Build history of the part. All positions in model axes, mm. Face numbers are marked on the shaded views. Round coordinates to 2 decimals unless told otherwise and drop trailing zeros. Loops run counter-clockwise (first coordinate to the right, second up) from the corner with the lowest first, then second, coordinate; pieces in that order, holes last. Notation, with made-up numbers: (-28, 55.25) - (8, 55.25) arc R37 ccw to (8, 91.25) - close; hole circle Ø4 at (-9, -22.75). An arc over 180 degrees is marked (long way). Use one line per item in the form item = value. Start each with the question number.
Q1. Mould opens along Z. For the marked faces 1, 2 and 3 say: released by +Z, released by -Z, zero draft, split by the parting line, or undercut.
Q2. Drill centre lines: line 1 (Z direction, x = 18.75, y = 0); line 2 (Z direction, x = 11, y = 4.75); line 3 (X direction, y = -10.5, z = -2.5). Where is each one in solid material? Low to high.
Q3. Pin check, flat tips, straight feed: pin 1 (4 mm diameter, centred on x = 5.5, z = 3.5, fed in from +Y); pin 2 (1 mm diameter, centred on x = 21, y = 0.5, fed in from -Z); pin 3 (4 mm diameter, centred on x = 5.5, y = -3.5, fed in from +Z); pin 4 (7.5 mm diameter, centred on y = -6, z = -2.5, fed in from +X). Stop position of each tip, or through.
Q4. Saw through at A-A (z = 0). Give the cut face in (x, y), then the cut area to 3 significant figures.
Q5. Saw through at C-C (x = 11.5). Give the cut face in (y, z).
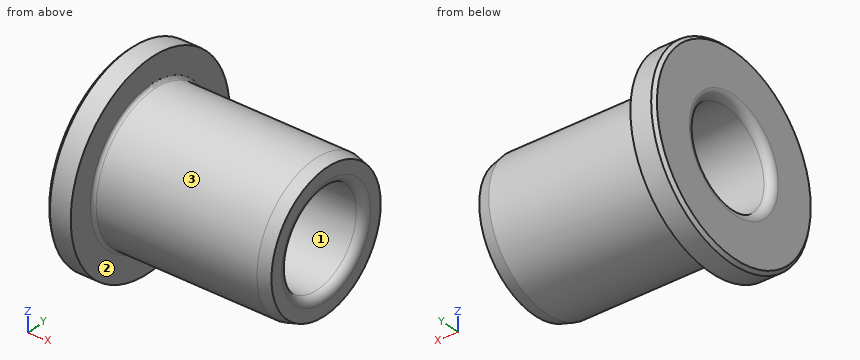
Autodesk Inventor part; units mm, degrees
ref_plane "YZ Plane" through (0, 0, 0) normal (1, 0, 0) x (0, 1, 0)
ref_plane "XZ Plane" through (0, 0, 0) normal (0, 1, 0) x (-1, 0, 0)
ref_plane "XY Plane" through (0, 0, 0) normal (0, 0, 1) x (1, 0, 0)
sketch "Sketch_1" plane through (0, 0, 0) normal (0, 0, 1) x (1, 0, 0)
  line L0 (25, 0) -> (0, 0)
  line L1 (0, 12.1) -> (0, 7)
  arc A0 (0, 7) -> (1, 6) centre (1, 7) ccw
  line L2 (1, 6) -> (24, 6)
  arc A1 (24, 6) -> (25, 7) centre (24, 7) ccw
  line L3 (25, 7) -> (25, 8.5981)
  line L4 (25, 8.5981) -> (23.5, 9)
  line L5 (23.5, 9) -> (3.4, 9)
  arc A2 (3, 9.4) -> (3.4, 9) centre (3.4, 9.4) ccw
  line L6 (3, 9.4) -> (3, 12.5)
  line L7 (3, 12.5) -> (0.4, 12.5)
  line L8 (0.4, 12.5) -> (0, 12.1)
revolve "Revolution1" add sketch "Sketch_1" angle 360 about axis through (25, 0, 0) along (1, 0, 0)
properties part number "SHFZ12_25"
Report:
q1.face_1 = undercut
q1.face_2 = zero draft
q1.face_3 = split by the parting line
q2.line_1 = -9 to -6, 6 to 9
q2.line_2 = -7.64 to -3.67, 3.67 to 7.64
q2.line_3 = 0 to 3
q3.pin_1 = 8.87
q3.pin_2 = -9
q3.pin_3 = 8.87
q3.pin_4 = 25
q4.outline = (0, -12.1) - (0.4, -12.5) - (3, -12.5) - (3, -9.4) arc R0.4 cw to (3.4, -9) - (23.5, -9) - (25, -8.6) - (25, -7) arc R1 ccw to (24, -6) - (1, -6) arc R1 ccw to (0, -7) - close; (0, 7) arc R1 ccw to (1, 6) - (24, 6) arc R1 ccw to (25, 7) - (25, 8.6) - (23.5, 9) - (3.4, 9) arc R0.4 cw to (3, 9.4) - (3, 12.5) - (0.4, 12.5) - (0, 12.1) - close
q4.area = 169 mm²
q5.outline = circle Ø18 at (0, 0); hole circle Ø12 at (0, 0)
